Input: dimensioned drawing with shaded views. Units: mm. Origin: part minimum x, y, z. Coordinates: 2 decimals unless noted, no trailing zeros. Order: outer loops, then holes, each group sorted by start corner. A loop starts at its lowest first (then second) coordinate and runs counter-clockwise, first axis right, second up. Notation, with made-up numbers: (-21, 35.25) - (38, 35.25) arc R13 ccw to (38, 45.25) - close; hole circle Ø8 at (26, 88.5). An arc over 180 degrees is marked (long way). Answer as CSV lines item,"result". Start each with the question number.
Item 1: Material intervals for line 1 along Z through (x, y) = (12.5, 5.5); line 2 along Z through (x, y) = (3, 20); line 3 along X through (y, z) = (9, 0.75), sorted ascending.
Item 2: First-contact query: pin 1 (1.1 mm diameter, centred on x = 15.5, z = 5.5, fed in from +Y); pin 2 (0.8 mm diameter, centred on x = 9.5, z = 5.5, fed in from +Y); pin 3 (1 mm diameter, centred on y = 19, z = 3, fed in from -X). Flat tips, straight axial feed; report the tip coordinate or a pass-through.
Item 3: Section B-B (z = 1.5). Output: boundary loops of the cut face in (x, y).
Item 4: Section C-C (z = 3.25). Output: boundary loops of the cut face in (x, y) (3 decimals), and give its area (3 significant figures).
Item 5: Section A-A (x = 15). Output: boundary loops of the cut face in (y, z).
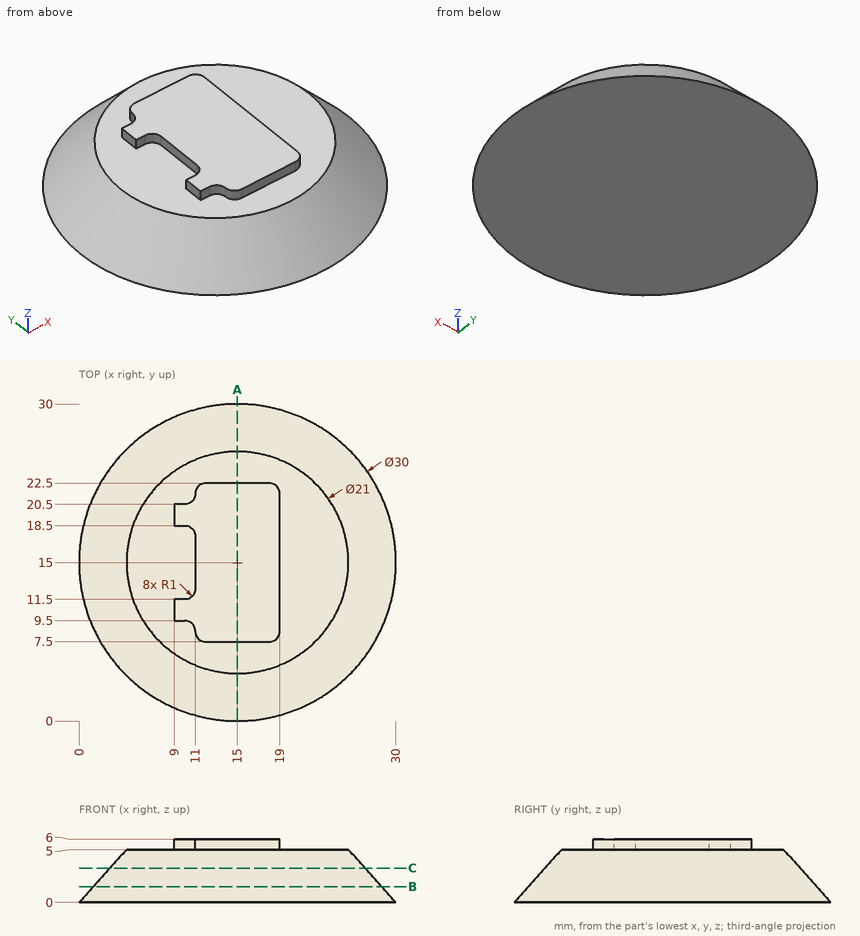
Determined:
1,line 1,"z = 0 to 5"
1,line 2,"z = 0 to 2.22"
1,line 3,"x = 1.99 to 28.01"
2,pin 1,"stops at y = 25.53"
2,pin 2,"stops at y = 20.5"
2,pin 3,"stops at x = 2.87"
3,outline,"circle Ø27.3 at (15, 15)"
4,outline,"circle Ø24.15 at (15, 15)"
4,area,"458 mm^2"
5,outline,"(0, 0) - (30, 0) - (25.5, 5) - (22.5, 5) - (22.5, 6) - (7.5, 6) - (7.5, 5) - (4.5, 5) - close"
